Geometry: final body of the model. Coordinates: model frame, mm. Face numbers are marked on the shaded views. Give positions to 0.01 mm unless a question says otherwise; leave off trailing zeros. Order: outer loops, then holes, each group sorted by start corner. A loop starts at its lowest first (then second) coordinate and runs counter-clockwise, first axis right, second up. Notation, with made-up numbers: (33, -32.75) - (65, -32.75) arc R19 ccw to (65, -8.75) - close; hole circle Ø4 at (3.25, 58). An arc over 180 degrees is marked (long way). One line per question, with ' | ' between items. Start each with the question number.
from build123d import *

# Parameters (mm, degrees)
SKETCH_1_R      = 0.4
EXTRUDE_2_DEPTH = 3
SKETCH_2_R      = 0.4
EXTRUDE_3_DEPTH = 3
SKETCH_3_R      = 6.25
EXTRUDE_4_DEPTH = 35


with BuildPart() as part:
    # Sketch 1 → Extrude 2 (new body)
    with BuildSketch(Plane(origin=(0, 0, 0), x_dir=(1, 0, 0), z_dir=(0, 1, 0))):
        with Locations((-2.5, 0)):
            Circle(SKETCH_1_R)
    extrude(amount=-EXTRUDE_2_DEPTH)



with BuildPart() as body_2:
    # Sketch 2 → Extrude 3 (new body)
    with BuildSketch(Plane(origin=(0, 0, 0), x_dir=(1, 0, 0), z_dir=(0, 1, 0))):
        with Locations((2.5, 0)):
            Circle(SKETCH_2_R)
    extrude(amount=-EXTRUDE_3_DEPTH)


with BuildPart() as part_1:
    add(part.part)

    add(body_2.part)  # Extrude 4 merges body 2
    # Sketch 3 → Extrude 4 (add)
    with BuildSketch(Plane(origin=(0, 0, 0), x_dir=(1, 0, 0), z_dir=(0, 1, 0))):
        Circle(SKETCH_3_R)
    extrude(amount=EXTRUDE_4_DEPTH)


solid = part_1.part
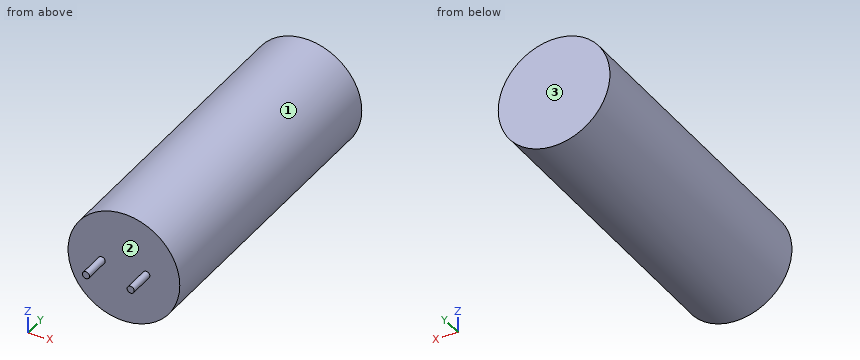
(1) Cut plane C-C, the plane y = 31. Return the cut outline in (x, z), plus the area to 3 significant figures.
(2) Pull-direction query (Y, two-part tool) for the marked faces 1, 2 and 3; classes: +Y half, -Y half, draft (parallel to the pull), parting line (faces both ways), or undercut.
(3) Cut plane A-A, the plane z = 0. Return the cut outline in (x, y), plus the area to 3 significant figures.
(4) Material intervals for line 1 along Y through (x, z) = (1.5, 0.25); line 2 along Z through (x, y) = (-0.25, 2.5) (3 decimals); line 3 along Z through (x, y) = (2.25, 32.5), sorted ascending. Write a range as from..to.
(5) Cut plane D-D, the plane x = 0. Return the cut outline in (y, z), plus the area to 4 significant figures.
(6) Contact query for flat-ended pins moving along their axis: P1, Ø2, axis at x = -4.5, z = 3.5, coming from the -Y side; P2, Ø1.5, axis at y = 5.5, z = -4.5, coming from the -X side; P3, Ø3, axis at x = -2, y = 15, coming from the -Z side. Output: stop coordinate, or through.
(7) Cut plane B-B, the plane x = -5. Return the cut outline in (y, z).
Results are:
1) outline: circle Ø12.5 at (0, 0) | area: 123 mm2
2) face 1: draft | face 2: -Y half | face 3: +Y half
3) outline: (-6.25, 0) - (-2.9, 0) - (-2.9, -3) - (-2.1, -3) - (-2.1, 0) - (2.1, 0) - (2.1, -3) - (2.9, -3) - (2.9, 0) - (6.25, 0) - (6.25, 35) - (-6.25, 35) - close | area: 442 mm2
4) line 1: 0..35 | line 2: -6.245..6.245 | line 3: -5.83..5.83
5) outline: (0, -6.25) - (35, -6.25) - (35, 6.25) - (0, 6.25) - close | area: 437.5 mm2
6) P1: y = 0 | P2: x = -5 | P3: z = -6.23
7) outline: (0, -3.75) - (35, -3.75) - (35, 3.75) - (0, 3.75) - close
